Geometry: final body of the model. Coordinates: model frame, mm. Face numbers are marked on the shaded views. A direction names the side the tool comes from. Give positions to 0.01 mm unless a question says otherwise; leave off trailing zeros. Write each loop counter-clockwise with the first axis right and the second up, starting at its lowest first coordinate (ties: lowest second). Pieces come first, ordered by that corner, then holes.
Q1. Section C-C (z = 4.55). Return the cut outline in (x, y).
Q2. Section B-B (x = -1.75). State how many separate pieces and enclosed holes the cut face has, plus the area to 3 significant figures.
Q3. Section A-A (z = 2.85). Return the cut outline in (x, y), plus the area to 3 significant figures.
Q4. Mould query, pull axis X, two halves, no side actions, for the marked faces 1, 2, 3 and 4. Classes: +X half, -X half, draft (parallel to the pull), parting line (faces both ways), or undercut.
Q5. Reachability of the marked faces 5 and 6 from +Z, -Z, +X, -X, +Y, -Y: full face, straight path, thin tool, end or side. Return the list, or none.
Q6. Line query: line 1 (Y direction, x = -2.75, z = 1.2); line 2 (X direction, y = -1.05, z = 2.85); line 3 (X direction, y = -0.85, z = 4). Output: solid intervals per line, ascending.
Q7. Pin query (flat end, axial travel): pin 1 Ø1.6 at (x, y) = (1.5, 0) entering from +Z; pin 2 Ø1.7 at (x, z) = (1.98, 4.31) entering from +Y. Return the tip coordinate at first contact, or that it passes through.
from build123d import *

# Parameters (mm, degrees)
F1_DEPTH = 5.755
F2_R     = 0.75
F3_DEPTH = 25
F4_DEPTH = 1


with BuildPart() as f1:
    # F0 (on Top) → F1 (new body)
    with BuildSketch(Plane.XY):
        Polygon((-3.7, -2.15), (3.7, -2.15), (3.7, -0.5), (3.2, -0.5), (3.2, -1.65), (-3.2, -1.65), (-3.2, -1), (-0.924631, -1), (-0.924631, -0.5), (-3.7, -0.5), align=None)
        Polygon((3.2, 0.5), (3.7, 0.5), (3.7, 2.15), (-3.7, 2.15), (-3.7, 0.5), (-0.924631, 0.5), (-0.924631, 1), (-3.2, 1), (-3.2, 1.65), (3.2, 1.65), align=None)
    extrude(amount=F1_DEPTH)

    # F2 (on face) → F3 (cut)
    with BuildSketch(Plane.XZ.offset(2.15)):
        with Locations((1.980075, 4.308214)):
            Circle(F2_R)
        with Locations((1.980075, 1.829074)):
            Circle(F2_R)
        with Locations((-2.004864, 1.798502)):
            Circle(F2_R)
    extrude(amount=-F3_DEPTH, mode=Mode.SUBTRACT)

    # F0 (on Top) → F4 (join)
    with BuildSketch(Plane.XY):
        Polygon((3.2, -0.5), (3.7, -0.5), (3.7, 0.5), (3.2, 0.5), (3.2, 1.65), (-3.2, 1.65), (-3.2, 1), (-0.924631, 1), (-0.924631, 0.5), (-0.924631, -0.5), (-0.924631, -1), (-3.2, -1), (-3.2, -1.65), (3.2, -1.65), align=None)
    extrude(amount=F4_DEPTH)


solid = f1.part
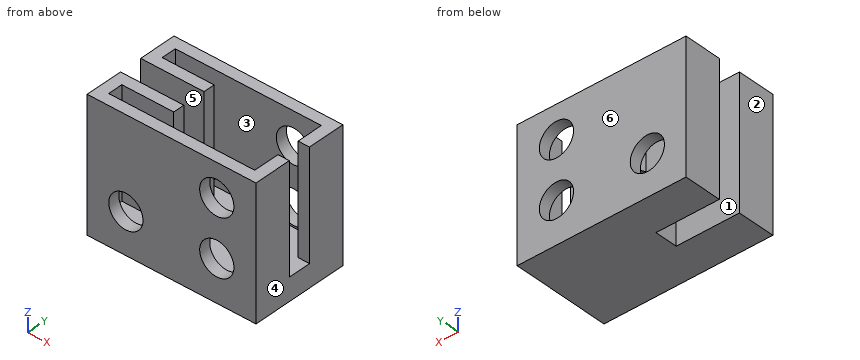
Computed:
1. outline: (-3.7, -2.15) - (1.27, -2.15) - (1.27, -1.65) - (-3.2, -1.65) - (-3.2, -1) - (-0.92, -1) - (-0.92, -0.5) - (-3.7, -0.5) - close; (-3.7, 0.5) - (-0.92, 0.5) - (-0.92, 1) - (-3.2, 1) - (-3.2, 1.65) - (1.27, 1.65) - (1.27, 2.15) - (-3.7, 2.15) - close; (2.69, -2.15) - (3.7, -2.15) - (3.7, -0.5) - (3.2, -0.5) - (3.2, -1.65) - (2.69, -1.65) - close; (2.69, 1.65) - (3.2, 1.65) - (3.2, 0.5) - (3.7, 0.5) - (3.7, 2.15) - (2.69, 2.15) - close
2. separate pieces: 6
2. enclosed holes: 0
2. area: 9.99 mm2
3. outline: (-3.7, -2.15) - (3.7, -2.15) - (3.7, -0.5) - (3.2, -0.5) - (3.2, -1.65) - (-3.2, -1.65) - (-3.2, -1) - (-0.92, -1) - (-0.92, -0.5) - (-3.7, -0.5) - close; (-3.7, 0.5) - (-0.92, 0.5) - (-0.92, 1) - (-3.2, 1) - (-3.2, 1.65) - (3.2, 1.65) - (3.2, 0.5) - (3.7, 0.5) - (3.7, 2.15) - (-3.7, 2.15) - close
3. area: 12.0 mm2
4. face 1: draft
4. face 2: -X half
4. face 3: undercut
4. face 4: +X half
5. face 5: +Z, -Z, -X
5. face 6: +Z, -Z, +X, -X, +Y
6. line 1: y = -2.15 to -1.65, -1 to -0.5, 0.5 to 1, 1.65 to 2.15
6. line 2: x = -3.7 to -3.2, 3.2 to 3.7
6. line 3: x = -3.7 to -0.92, 3.2 to 3.7
7. pin 1: stops at z = 1
7. pin 2: stops at y = 2.15
